Check sheet for the drawn part. Datum: minimum x, y, z corner. Units: mm. Give positions to 0.01 mm unless a question says otherwise; leave off trailing zeros. Write each loop counter-clockwise with the first axis right and the second up, starting at its lowest first coordinate (ties: lowest second). Pieces come first, ordered by that corner, then holes. Notation, with made-up numbers: (47.5, 2.5) -> (88.5, 2.5) arc R27 cw to (88.5, 25.5) -> close; hole circle Ø10 at (32.25, 82.25). An arc over 180 degrees is marked (long way). Write item = value, one per line. Start each with the question number.
1. Cross-section at D-D, the plane z = 15.5. Record the cut outline in (x, y), plus the area to 3 significant figures.
2. Mould release check, pull along X, two halves, no side actions. Record for the marked faces 1 and 2: pulls with the +X half, pulls with the -X half, needs draft (parallel to the pull), parting line crosses it, or undercut.
3. Cross-section at A-A, the plane y = 1.4. Record the cut outline in (x, z).
4. Depth check by flat-ended pin: P1, Ø2, axis at y = 3.5, z = 12.5, coming from the -X side; P2, Ø3, axis at x = 14, z = 5.5, coming from the -Y side; P3, Ø4, axis at x = 11.5, z = 9.5, coming from the -Y side. Enter the tip coordinate at first touch or a pass-through.
5. Cross-section at B-B, the plane x = 14. Record the cut outline in (y, z).
6. Thickness scan on line 1 along X through (y, z) = (3.65, 9); line 2 along Z through (x, y) = (14, 3.15); line 3 along X through (y, z) = (2, 9.75). Record the ranges inside material, lowest first.
7. Cross-section at C-C, the plane y = 3.4. Record the cut outline in (x, z).
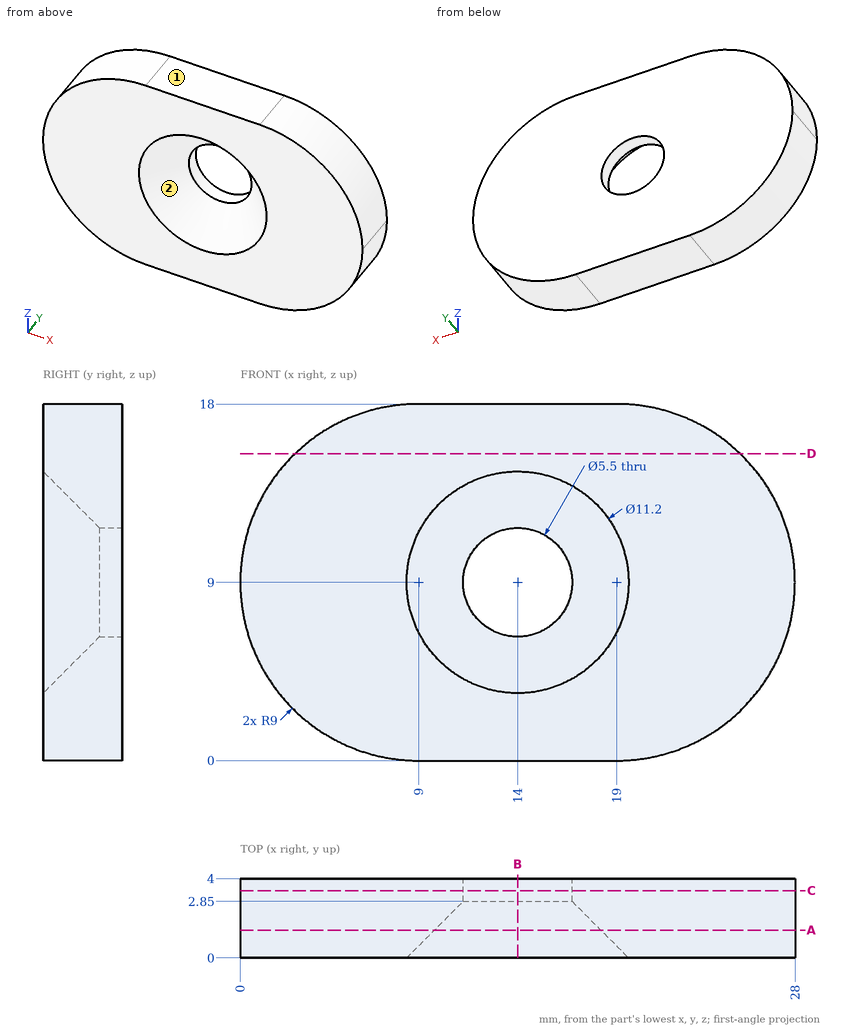
Answers:
q1.outline = (2.78, 0) -> (25.22, 0) -> (25.22, 4) -> (2.78, 4) -> close
q1.area = 89.8 mm^2
q2.face_1 = needs draft
q2.face_2 = undercut
q3.outline = (9, 0) -> (19, 0) arc R9 ccw to (19, 18) -> (9, 18) arc R9 ccw to start; hole circle Ø8.4 at (14, 9)
q4.P1 = 0.35
q4.P2 = 0.6
q4.P3 = 1.05
q5.outline = (0, 0) -> (4, 0) -> (4, 6.25) -> (2.85, 6.25) -> (0, 3.4) -> close; (0, 14.6) -> (2.85, 11.75) -> (4, 11.75) -> (4, 18) -> (0, 18) -> close
q6.line_1 = 0 to 11.25, 16.75 to 28
q6.line_2 = 0 to 6.25, 11.75 to 18
q6.line_3 = 0.03 to 10.48, 17.52 to 27.97
q7.outline = (9, 0) -> (19, 0) arc R9 ccw to (19, 18) -> (9, 18) arc R9 ccw to start; hole circle Ø5.5 at (14, 9)
